Read the model definition and answer for the solid it produces. Units are mm, in the model's axes. Face numbers are marked on the shaded views. A direction names the side the tool comes from. Round coordinates to 2 decimals unless told otherwise and drop trailing zeros. Order: outer loops, then holes, each group sorted by start corner. A loop starts at its lowest first (then second) coordinate and runs counter-clockwise, first axis right, second up. Notation, with made-up numbers: (0.5, -23) -> (12.5, -23) arc R17 ccw to (12.5, -18) -> close; hole circle Ø9 at (-19.5, 35). An arc over 180 degrees is marked (long way). One line per item, written item: value. Start each with the question number.
1. Consider line 1 (Y direction, x = 64, z = 42.5); line 2 (Y direction, x = 14.5, z = 56.5); line 3 (Z direction, x = 91, y = -16) (3 decimals). Determine where each line is inside the solid, lowest interval first.
2. For the marked faces 1, 2, 3 and 4, determine the directions among +Z, -Z, +X, -X, +Y, -Y from which every point of the face is accessible in a straight line to the end or side of a thin tool.
3. Section C-C (y = 39) is taken. Give the vertices of the cut face in (x, z) (3 decimals).
4. Section B-B (y = 21.5) is taken. Give the vertices of the cut face in (x, z) (3 decimals).
5. Flat-ended cylindrical pins translate along their axes: pin 1 Ø12 at (x, z) = (49.5, 24) entering from +Y; pin 2 Ø10 at (x, z) = (40, 15.5) entering from +Y; pin 3 Ø8 at (x, y) = (76, 14) entering from -Z; pin 4 Ø3 at (x, y) = (4.5, 6) entering from +Z. Find the tip coordinate at first contact, or state that the pin passes through.
6. Section A-A (y = -11) is taken. Give the vertices of the cut face in (x, z) (3 decimals), then the cut area to 3 significant figures.
from build123d import *

# Parameters (mm, degrees)
F1_DEPTH = 63.5
F2_DEPTH = 25.4
F3_DEPTH = 7.9375
F4_DEPTH = 25.4
F6_R     = 6.35


with BuildPart() as f1:
    # F0 (on Front) → F1 (new body, symmetric)
    with BuildSketch(Plane.XZ):
        Polygon((41.275, -9.525), (41.275, 9.525), (22.225, 9.525), (-41.275, 9.525), (-41.275, -9.525), align=None)
    extrude(amount=F1_DEPTH, both=True)

    # F0 (on Front) → F2 (join, symmetric)
    with BuildSketch(Plane.XZ):
        with BuildLine():
            Line((22.225, 9.525), (41.275, 9.525))
            Line((41.275, 9.525), (41.275, 27.934134))
            ThreePointArc((41.275, 27.934134), (44.165769, 37.067884), (51.785284, 42.8752))
            Line((51.785284, 42.8752), (52.741684, 42.8752))
            Line((52.741684, 42.8752), (52.741684, 61.9252))
            Line((52.741684, 61.9252), (49.12734, 61.9252))
            ThreePointArc((49.12734, 61.9252), (29.764356, 49.608592), (22.225, 27.934134))
            Line((22.225, 27.934134), (22.225, 9.525))
        make_face()
    extrude(amount=F2_DEPTH, both=True)

    # F0 (on Front) → F3 (join, symmetric)
    with BuildSketch(Plane.XZ):
        with BuildLine():
            Line((-41.275, 9.525), (22.225, 9.525))
            Line((22.225, 9.525), (22.225, 27.934134))
            ThreePointArc((22.225, 27.934134), (29.764356, 49.608592), (49.12734, 61.9252))
            add(Edge.make_bspline(
                [(-41.275, 9.525), (-40.009573, 46.556816), (13.483403, 60.000081), (49.12734, 61.9252)],
                knots=[0, 0, 0, 0, 104.490976, 104.490976, 104.490976, 104.490976], degree=3))
        make_face()
    extrude(amount=F3_DEPTH, both=True)

    # F0 (on Front) → F4 (join, symmetric)
    with BuildSketch(Plane.XZ):
        Polygon((52.741684, 61.9252), (52.741684, 42.8752), (52.741684, 38.1), (78.141684, 38.1), (78.141684, 61.9252), align=None)
    extrude(amount=F4_DEPTH, both=True)

    # F0 (on Front) → F5 (revolve)
    with BuildSketch(Plane.XZ):
        Polygon((78.141684, 66.675), (78.141684, 61.9252), (78.141684, 38.1), (103.541684, 38.1), (103.541684, 66.675), align=None)
    revolve(axis=Axis((78.141684, 0, 52.3875), (0, 0, 1)))

    # F6
    f6_edges = [f1.edges().sort_by_distance(p)[0] for p in [
        (41.275, -63.5, 0),
        (-41.275, -63.5, 0),
        (-41.275, 63.5, 0),
        (41.275, 63.5, 0),
    ]]
    fillet(f6_edges, radius=F6_R)


solid = f1.part
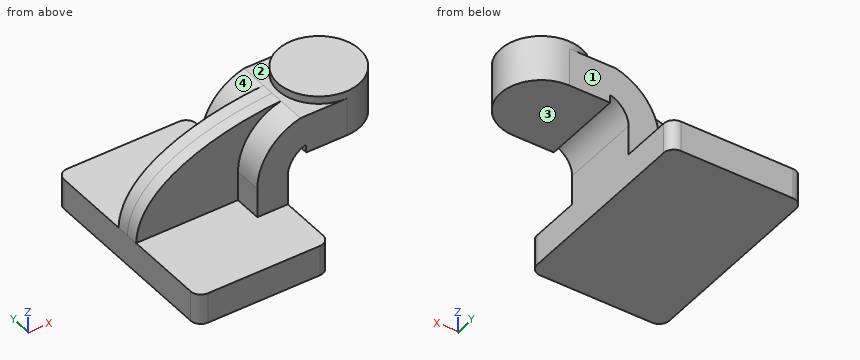
Answer:
1. line 1: -25.4 to 25.4
1. line 2: -7.94 to 7.94
1. line 3: 38.1 to 66.675
2. face 1: +Z, +X, -X, +Y
2. face 2: +Z, -X
2. face 3: -Z, +X, +Y, -Y
2. face 4: +Z, -X, +Y
3. outline: (-41.275, -9.525) -> (41.275, -9.525) -> (41.275, 9.525) -> (-41.275, 9.525) -> close
4. outline: (-41.275, -9.525) -> (41.275, -9.525) -> (41.275, 27.934) arc R15.875 cw to (51.785, 42.875) -> (52.742, 42.875) -> (52.742, 38.1) -> (91.666, 38.1) -> (91.666, 66.675) -> (64.617, 66.675) -> (64.617, 61.925) -> (49.127, 61.925) arc R34.925 ccw to (22.225, 27.934) -> (22.225, 9.525) -> (-41.275, 9.525) -> close
5. pin 1: through
5. pin 2: y = 25.4
5. pin 3: z = 38.1
5. pin 4: z = 54.51
6. outline: (-41.275, -9.525) -> (41.275, -9.525) -> (41.275, 27.934) arc R15.875 cw to (51.785, 42.875) -> (52.742, 42.875) -> (52.742, 38.1) -> (101.036, 38.1) -> (101.036, 66.675) -> (55.247, 66.675) -> (55.247, 61.925) -> (49.127, 61.925) arc R34.925 ccw to (22.225, 27.934) -> (22.225, 9.525) -> (-41.275, 9.525) -> close
6. area: 3,970 mm^2
